```python
from build123d import *

# Parameters (mm, degrees)
SKETCH1_R           = 2
BOSS_EXTRUDE1_DEPTH = 2


with BuildPart() as part:
    # Sketch1 → Boss-Extrude1 (new body)
    with BuildSketch(Plane.XY):
        with BuildLine():
            Line((-15.236964255, 46.840062703), (-15.236964255, -18.159937297))
            Line((-15.236964255, -18.159937297), (35.163035745, -18.159937297))
            Line((35.163035745, -18.159937297), (35.163035745, 7.240062703))
            Line((35.163035745, 7.240062703), (22.463035745, 7.240062703))
            ThreePointArc((22.463035745, 7.240062703), (14.841940785, 9.199641421), (9.763035745, 15.210112346))
            Line((9.763035745, 15.210112346), (9.763035745, 46.840062703))
            Line((9.763035745, 46.840062703), (-15.236964255, 46.840062703))
        make_face()
        with Locations((-2.736964255, -9.659937297)):
            Circle(SKETCH1_R, mode=Mode.SUBTRACT)
        with Locations((-2.736964255, 38.340062703)):
            Circle(SKETCH1_R, mode=Mode.SUBTRACT)
    extrude(amount=BOSS_EXTRUDE1_DEPTH)


solid = part.part
```
Check sheet for the modelled part. Datum: model origin and axes. Units: mm. A direction names the side the tool comes from. Round coordinates to 2 decimals unless told otherwise and drop trailing zeros. Order: outer loops, then holes, each group sorted by start corner. A loop starts at its lowest first (then second) coordinate and runs counter-clockwise, first axis right, second up. Notation, with made-up numbers: (66.5, -34.75) - (71.5, -34.75) arc R27 cw to (71.5, -3.75) - close; hole circle Ø10 at (47, 52). An arc over 180 degrees is marked (long way). Write item = value, one per line.
Q1. Section check B-B (y = 30). Record the boundary of the cut face in (x, z).
Computed:
outline = (-15.24, 0) - (9.76, 0) - (9.76, 2) - (-15.24, 2) - close
Q2. Go/stop test with flat-tipped pins: pin 1 (1 mm diameter, centred on y = 30.5, z = 1.5, fed in from +X); pin 2 (3.5 mm diameter, centred on x = -2.74, y = -9.66, fed in from -Z). Record where each tip stops, or that it passes through.
Computed:
pin_1 = 9.76
pin_2 = through
Q3. Thickness scan on line 1 along X through (y, z) = (40.5, 0.2); line 2 along X through (y, z) = (-10, 0.55); line 3 along Y through (x, z) = (31.5, 1.85). Record the ranges inside material, lowest first.
Computed:
line_1 = -15.24 to 9.76
line_2 = -15.24 to -4.71, -0.77 to 35.16
line_3 = -18.16 to 7.24
Q4. Section check C-C (x = 17.5). Record the boundary of the cut face in (y, z), and give its area (3 significant figures).
Computed:
outline = (-18.16, 0) - (7.93, 0) - (7.93, 2) - (-18.16, 2) - close
area = 52.2 mm^2
Q5. Tool access check on faces 1 (the face through (-3, 46.84, 1)), 2 (the face through (9.763, 31, 1)). Record the directions out of +Z, -Z, +X, -X, +Y, -Y that give a thin tool (end or side, any length) a straight path to the whole face; none if there is none.
Computed:
face_1 = +Z, -Z, +X, -X, +Y
face_2 = +Z, -Z, +X, +Y
Q6. Draft check along X on faces 3 (the face through (-3.171, 36.388, 0.986)), 4 (the face through (-4.21, -8.31, 0.99)), 5 (the face through (4, 8, 0)), 6 (the face through (-15.237, 15, 1)). Enter one of: pulls with the +X half, pulls with the -X half, needs draft (parallel to the pull), parting line crosses it, or undercut.
Computed:
face_3 = undercut
face_4 = undercut
face_5 = needs draft
face_6 = pulls with the -X half
Q7. Section check A-A (z = 1.2). Record the boundary of the cut face in (x, y), and give its area (3 significant figures).
Computed:
outline = (-15.24, -18.16) - (35.16, -18.16) - (35.16, 7.24) - (22.46, 7.24) arc R12.95 cw to (9.76, 15.21) - (9.76, 46.84) - (-15.24, 46.84) - close; hole circle Ø4 at (-2.74, -9.66); hole circle Ø4 at (-2.74, 38.34)
area = 2,270 mm^2
